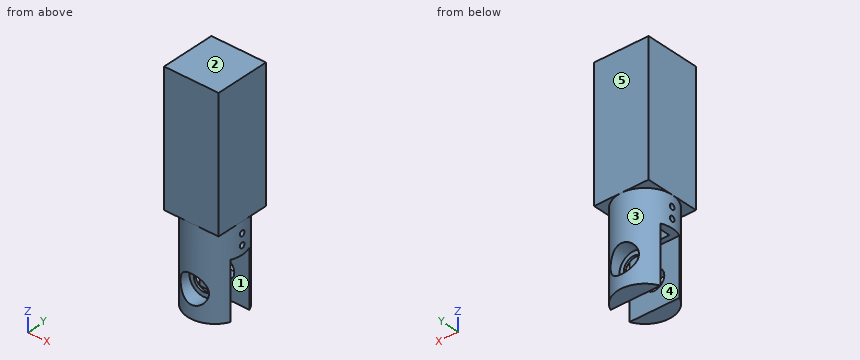
from build123d import *

# Parameters (mm, degrees)
SKETCH_1_R               = 12.5
EXTRUDE_1_DEPTH          = 100
CUT_EXTRUDE_START        = -26
CUT_EXTRUDE_1_DEPTH      = 26
CUT_EXTRUDE_2_DEPTH      = 34
CUT_EXTRUDE_2_DEPTH_BACK = 36.534771414
SKETCH_3_R               = 4.5
SKETCH_6_R               = 6.5
CUT_EXTRUDE_5_DEPTH      = 16
SKETCH_7_W               = 18
SKETCH_7_H               = 5
CUT_EXTRUDE_6_DEPTH      = 13
SKETCH_9_R               = 1.25
CUT_EXTRUDE_7_DEPTH      = 44
SKETCH_10_W              = 25
SKETCH_10_H              = 25
EXTRUDE_2_DEPTH          = 60


with BuildPart() as part:
    # 스케치1 → 보스-돌출1 (new body)
    with BuildSketch(Plane.XY):
        Circle(SKETCH_1_R)
    extrude(amount=-EXTRUDE_1_DEPTH)

    # 스케치2 → 컷-돌출1 (cut)
    with BuildSketch(Plane(origin=(0, 0, -100), x_dir=(-1, 0, 0), z_dir=(0, 0, -1)).offset(CUT_EXTRUDE_START)):
        with BuildLine():
            Line((11.456439237, 5), (-11.456439237, 5))
            ThreePointArc((-11.456439237, 5), (-12.5, 0), (-11.456439237, -5))
            Line((-11.456439237, -5), (11.456439237, -5))
            ThreePointArc((11.456439237, -5), (12.5, 0), (11.456439237, 5))
        make_face()
    extrude(amount=CUT_EXTRUDE_1_DEPTH, mode=Mode.SUBTRACT)

    # 스케치3 → 컷-돌출2 (cut, two sides: drawn at the far end of the back side and taken through both)
    with BuildSketch(Plane(origin=(0, 0, 0), x_dir=(1, 0, 0), z_dir=(0, 1, 0)).offset(-CUT_EXTRUDE_2_DEPTH_BACK)):
        with Locations(Location((0, 87.5, 0), (0, 0, 90))):
            Circle(SKETCH_3_R)
    extrude(amount=CUT_EXTRUDE_2_DEPTH + CUT_EXTRUDE_2_DEPTH_BACK, mode=Mode.SUBTRACT)

    # 스케치6 → 컷-돌출5 (cut)
    with BuildSketch(Plane(origin=(0, 6, 0), x_dir=(1, 0, 0), z_dir=(0, 1, 0))):
        with Locations(Location((0, 87.5, 0), (0, 0, 90))):
            Circle(SKETCH_6_R)
    cut_extrude_5 = extrude(amount=CUT_EXTRUDE_5_DEPTH, mode=Mode.SUBTRACT)

    # 대칭 복사1: 컷-돌출5 across plane
    add(cut_extrude_5.mirror(Plane.ZX), mode=Mode.SUBTRACT)

    # 스케치7 → 컷-돌출6 (cut)
    with BuildSketch(Plane(origin=(0, 0, -74), x_dir=(-1, 0, 0), z_dir=(0, 0, -1))):
        Rectangle(SKETCH_7_W, SKETCH_7_H)
    extrude(amount=-CUT_EXTRUDE_6_DEPTH, mode=Mode.SUBTRACT)

    # 스케치9 → 컷-돌출7 (cut)
    with BuildSketch(Plane(origin=(12.5, 0, 0), x_dir=(0, 0, -1), z_dir=(1, 0, 0))):
        with Locations((70, 0)):
            Circle(SKETCH_9_R)
        with Locations((65, 0)):
            Circle(SKETCH_9_R)
    extrude(amount=-CUT_EXTRUDE_7_DEPTH, mode=Mode.SUBTRACT)

    # 스케치10 → 보스-돌출2 (add)
    with BuildSketch(Plane.XY):
        Rectangle(SKETCH_10_W, SKETCH_10_H)
    extrude(amount=-EXTRUDE_2_DEPTH)


solid = part.part
Geometry check sheet. Reference: the model listing, model coordinates, mm. Face numbers are marked on the shaded views. A direction names the side the tool comes from. Give positions to 0.01 mm unless a question says otherwise; leave off trailing zeros. Order: outer loops, then holes, each group sorted by start corner. A loop starts at its lowest first (then second) coordinate and runs counter-clockwise, first axis right, second up.
1) Draft check along Y on the marked faces 3, 4 and 5. Enter one of: released by +Y, released by -Y, zero draft, split by the parting line, or undercut.
Results are:
face 3: split by the parting line
face 4: undercut
face 5: released by +Y
2) Cross-section at C-C (z = -87.5). Record the boundary of the cut face in (x, y).
Results are:
outline: (-11.46, -5) arc R12.5 ccw to (-6.5, -10.68) - (-6.5, -6) - (-4.5, -6) - (-4.5, -5) - close; (-11.46, 5) - (-4.5, 5) - (-4.5, 6) - (-6.5, 6) - (-6.5, 10.68) arc R12.5 ccw to start; (4.5, -6) - (6.5, -6) - (6.5, -10.68) arc R12.5 ccw to (11.46, -5) - (4.5, -5) - close; (4.5, 5) - (11.46, 5) arc R12.5 ccw to (6.5, 10.68) - (6.5, 6) - (4.5, 6) - close
3) Gauge pin test, flat ends, axial feed: pin 1 (2 mm diameter, centred on y = -9.5, z = -72, fed in from +X); pin 2 (11.5 mm diameter, centred on x = 0, z = -87.5, fed in from +Y); pin 3 (2 mm diameter, centred on y = 5.5, z = -70, fed in from -X); pin 4 (6 mm diameter, centred on x = -8.5, z = -62, fed in from +Y). Record the tip position at first contact, or that the pin passes through.
Results are:
pin 1: stops at x = 9.17
pin 2: stops at y = 6
pin 3: stops at x = -11.66
pin 4: stops at y = 12.5
4) Cross-section at A-A (x = 3.25). Give the number of separate pieces and of enclosed holes in the cut face, then the cut area to 3 significant figures.
Results are:
separate pieces: 3
enclosed holes: 0
area: 1,990 mm2
5) Material ranges on probe 1 along Z at (x, y) = (-10.45, 0); probe 2 along Y at (x, z) = (11.45, -70); probe 3 along Z at (x, y) = (11.25, 7), recorded low to high.
Results are:
probe 1: z = -74 to -71.25, -68.75 to -66.25, -63.75 to 0
probe 2: y = -5.01 to -1.25, 1.25 to 5.01
probe 3: z = -60 to 0
6) Cross-section at B-B (z = -70). Record the boundary of the cut face in (x, y).
Results are:
outline: (-12.44, -1.25) arc R12.5 ccw to (12.44, -1.25) - (9, -1.25) - (9, -2.5) - (-9, -2.5) - (-9, -1.25) - close; (-12.44, 1.25) - (-9, 1.25) - (-9, 2.5) - (9, 2.5) - (9, 1.25) - (12.44, 1.25) arc R12.5 ccw to start
7) Tool access check on the marked faces 1 and 2. Record the directions out of +Z, -Z, +X, -X, +Y, -Y that give a thin tool (end or side, any length) a straight path to the whole face; none if there is none.
Results are:
face 1: -Z, +X, -X
face 2: +Z, +X, -X, +Y, -Y
